The figure shows three views and two pictorial views of one solid part (mm, origin at its lowest corner). Answer the questions. Coordinates: 2 decimals unless noted, no trailing zeros. Order: outer loops, then holes, each group sorted by start corner. A loop starts at its lowest first (then second) coordinate and runs counter-clockwise, first axis right, second up. Notation, with made-up numbers: M 71.25,25 L 87.25,25 A16 cw 87.25,55 Z; hole C 11,-9.5 d8. An arc over 180 degrees is marked long. Answer in a Markdown table with one row per item. Add a question column.
Item 1: Flat-ended cylindrical pins translate along their axes: pin 1 Ø4 at (x, z) = (6, 74) entering from +Y; pin 2 Ø3 at (x, z) = (7, 2) entering from -Y. Find the tip coordinate at first contact, or state that the pin passes through.
Item 2: The part is cut by section B-B (y = 1.5). Write down the section's boundary in (x, z).
Item 3: The part is cut by section C-C (y = 10.25). Write down the section's boundary in (x, z).
Item 4: Consider line 1 (Z direction, x = 12, y = 7.75); line 2 (Y direction, x = 2.5, z = 17); line 3 (X direction, y = 1.5, z = 43.5). Determine where each line is inside the solid, lowest interval first. Write a range as from..to.
Item 5: The part is cut by section A-A (x = 5.5). Write down the section's boundary in (y, z), then the cut area to 3 significant figures.
Item 6: The part is cut by section D-D (z = 61.5). Write down the section's boundary in (x, y).
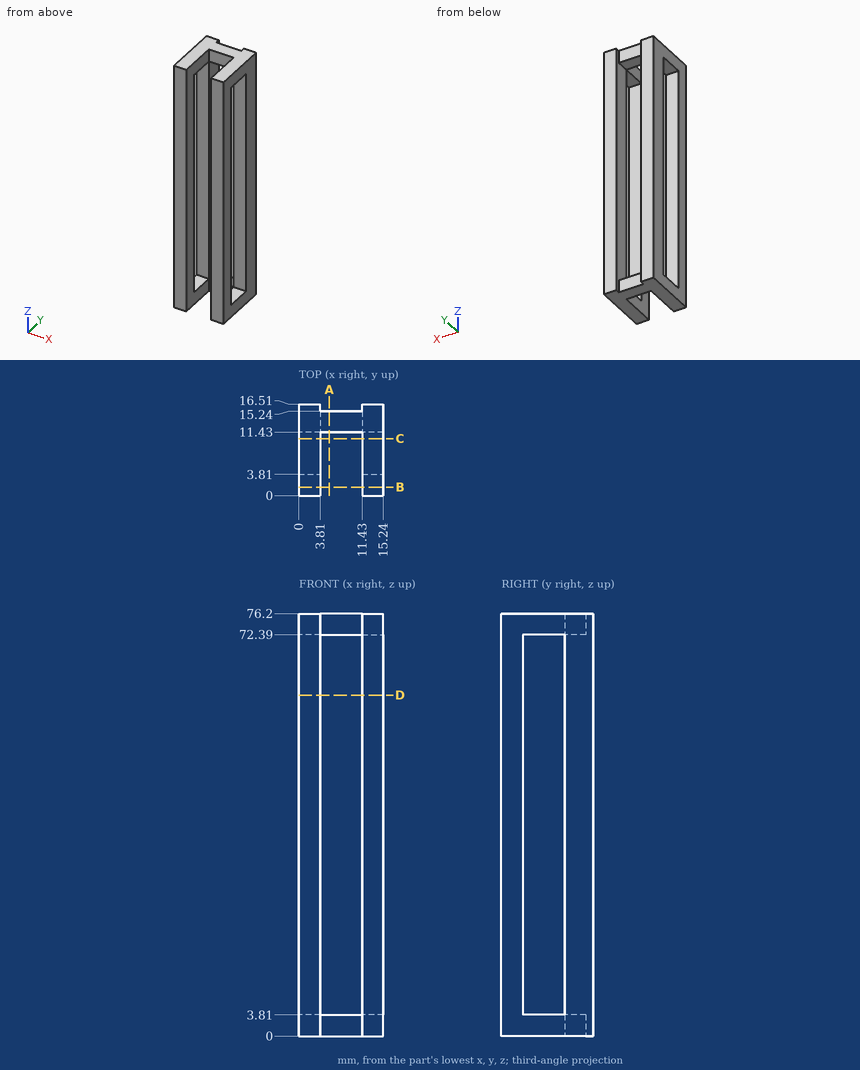
Reply:
| question | item | result |
|---|---|---|
| 1 | pin 1 | stops at y = 15.24 |
| 1 | pin 2 | stops at y = 11.43 |
| 2 | outline | M 0,0 L 3.81,0 L 3.81,76.2 L 0,76.2 Z; M 11.43,0 L 15.24,0 L 15.24,76.2 L 11.43,76.2 Z |
| 3 | outline | M 0,0 L 3.81,0 L 3.81,3.81 L 0,3.81 Z; M 0,72.39 L 3.81,72.39 L 3.81,76.2 L 0,76.2 Z; M 11.43,0 L 15.24,0 L 15.24,3.81 L 11.43,3.81 Z; M 11.43,72.39 L 15.24,72.39 L 15.24,76.2 L 11.43,76.2 Z |
| 4 | line 1 | z = 0..3.81, 72.39..76.2 |
| 4 | line 2 | y = 0..3.81, 11.43..16.51 |
| 4 | line 3 | x = 0..3.81, 11.43..15.24 |
| 5 | outline | M 11.43,0 L 15.24,0 L 15.24,3.81 L 11.43,3.81 Z; M 11.43,72.39 L 15.24,72.39 L 15.24,76.2 L 11.43,76.2 Z |
| 5 | area | 29.0 mm2 |
| 6 | outline | M 0,0 L 3.81,0 L 3.81,3.81 L 0,3.81 Z; M 0,11.43 L 3.81,11.43 L 3.81,16.51 L 0,16.51 Z; M 11.43,0 L 15.24,0 L 15.24,3.81 L 11.43,3.81 Z; M 11.43,11.43 L 15.24,11.43 L 15.24,16.51 L 11.43,16.51 Z |
